Source: CAD feature listing. Evaluate the final solid. Frame: model axes, mm. A direction names the side the tool comes from. Give positions to 0.01 mm unless a question says otherwise; leave off trailing zeros. Loops run counter-clockwise (first coordinate to the right, second up) from the corner with the lowest first, then second, coordinate; pieces in that order, holes last. Notation, with made-up numbers: M 34,-7.5 L 75,-7.5 A13 ccw 75,5.5 Z; hole C -20.5,-37 d5. An arc over 180 degrees is marked long. Answer in a Markdown table with one row per item.
Autodesk Inventor part; units mm, degrees
ref_plane "YZ Plane" through (0, 0, 0) normal (1, 0, 0) x (0, 1, 0)
ref_plane "XZ Plane" through (0, 0, 0) normal (0, 1, 0) x (-1, 0, 0)
ref_plane "XY Plane" through (0, 0, 0) normal (0, 0, 1) x (1, 0, 0)
sketch "Sketch1" plane through (0, 0, 0) normal (0, 0, 1) x (1, 0, 0)
  line L0 (0, 0) -> (79, 0)
  line L1 (79, 0) -> (79, 32)
  line L2 (79, 32) -> (0, 32)
  line L3 (0, 32) -> (0, 0)
  dimension "d0" = 79
  dimension "d1" = 32
extrude "Extrusion1" add sketch "Sketch1" along normal blind 26
sketch "Sketch2" plane through (0, 0, 26) normal (0, 0, 1) x (1, 0, 0)
  circle A0 centre (15, 16) radius 3
  line L0 (0, 32) -> (0, 0)
  line L1 (6.5, 24.75) -> (39.5, 24.75) construction
  line L2 (39.5, 24.75) -> (39.5, 7.25) construction
  line L3 (39.5, 7.25) -> (6.5, 7.25) construction
  line L4 (6.5, 7.25) -> (6.5, 24.75) construction
  circle A1 centre (6.5, 24.75) radius 1.5
  circle A2 centre (6.5, 7.25) radius 1.5
  circle A3 centre (39.5, 24.75) radius 1.5
  circle A4 centre (39.5, 7.25) radius 1.5
  point P0 (0, 16)
  point P1 (6.5, 16)
  dimension "d4" = 6
  dimension "d5" = 15
  dimension "d6" = 33
  dimension "d7" = 17.5
  dimension "d8" = 8.5
  dimension "d9" = 3
  dimension "d10" = 3
  dimension "d11" = 3
  dimension "d12" = 3
extrude "Extrusion2" add sketch "Sketch2" along normal blind 15 contours A0
extrude "Extrusion3" cut sketch "Sketch2" against normal blind 10 contours A1 | A2 | A3 | A4
properties part number "Motor"
1) Pin query (flat end, axial travel): pin 1 Ø1 at (x, y) = (42.5, 8.5) entering from +Z; pin 2 Ø1.5 at (x, y) = (39.5, 24.5) entering from +Z; pin 3 Ø6 at (y, z) = (10.5, 32.5) entering from -X. Return the tip coordinate at first contact, or that it passes through.
Reply:
| item | result |
|---|---|
| pin 1 | stops at z = 26 |
| pin 2 | stops at z = 16 |
| pin 3 | stops at x = 13.34 |
2) Pull-direction query (Y, two-part tool) for faces 3 (the flat face through (6, 7, 16)), 4 (the cylindrical face through (12.6, 17.8, 33.4)), 5 (the cylindrical face through (6.305, 26.237, 21.07)), 6 (the flat face through (0, 16, 13)); classes: released by +Y, released by -Y, zero draft, split by the parting line, or undercut.
Reply:
| item | result |
|---|---|
| face 3 | undercut |
| face 4 | split by the parting line |
| face 5 | undercut |
| face 6 | zero draft |
3) Section C-C, the plane y = 7.25. Return loops of the section in (x, z).
Reply:
| item | result |
|---|---|
| outline | M 0,0 L 79,0 L 79,26 L 41,26 L 41,16 L 38,16 L 38,26 L 8,26 L 8,16 L 5,16 L 5,26 L 0,26 Z |
4) Set-up query: faces 1 (the flat face through (39, 16, 0)), 2 (the cylindrical face through (38.39, 25.76, 21.07)). Return all of +Z, -Z, +X, -X, +Y, -Y with unobstructed straight access to the full face (end or side cutting, diameter ignored); none if empty.
Reply:
| item | result |
|---|---|
| face 1 | -Z, +X, -X, +Y, -Y |
| face 2 | +Z |
5) Section D-D, the plane z = 31. Return loops of the section in (x, y), then the cut area to 3 significant figures.
Reply:
| item | result |
|---|---|
| outline | C 15,16 d6 |
| area | 28.3 mm² |
6) Section A-A, the plane y = 16. Return loops of the section in (x, z).
Reply:
| item | result |
|---|---|
| outline | M 0,0 L 79,0 L 79,26 L 18,26 L 18,41 L 12,41 L 12,26 L 0,26 Z |
7) Section B-B, the plane x = 6.5. Return loops of the section in (y, z).
Reply:
| item | result |
|---|---|
| outline | M 0,0 L 32,0 L 32,26 L 26.25,26 L 26.25,16 L 23.25,16 L 23.25,26 L 8.75,26 L 8.75,16 L 5.75,16 L 5.75,26 L 0,26 Z |
8) Material intervals for L1, parallel to Y at x = 6.5, z = 22; L2, parallel to X at y = 24, z = 18; L3, parallel to X at y = 7, z = 20, sorted ascending.
Reply:
| item | result |
|---|---|
| L1 | y = 0 to 5.75, 8.75 to 23.25, 26.25 to 32 |
| L2 | x = 0 to 5.2, 7.8 to 38.2, 40.8 to 79 |
| L3 | x = 0 to 5.02, 7.98 to 38.02, 40.98 to 79 |
